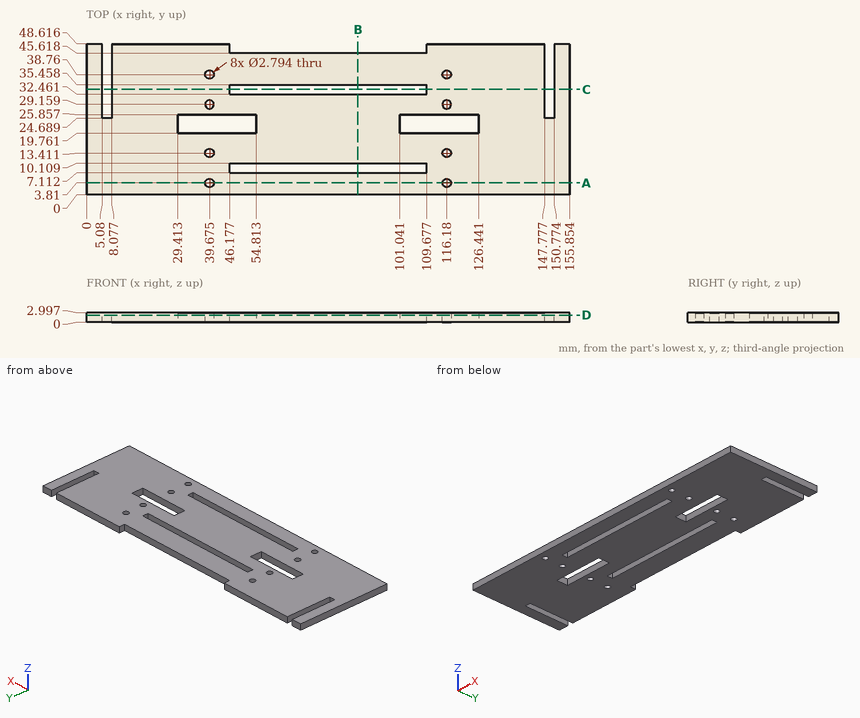
Check sheet for the drawn part. Datum: minimum x, y, z corner. Units: mm. Give positions to 0.01 mm unless a question says otherwise; leave off trailing zeros. Loops run counter-clockwise (first coordinate to the right, second up) from the corner with the lowest first, then second, coordinate; pieces in that order, holes last.
1) Sectioned sample at C-C, the plane y = 34. Enter the section's corners in (x, z) (1 decimal).
2) Depth check by flat-ended pin: pin 1 Ø1.5 at (x, z) = (149, 1.5) entering from +Y. Enter the tip coordinate at first touch or a pass-through.
3) Thickness scan on line 1 along X through (y, z) = (26, 2.6) (1 decimal); line 2 along Y through (x, z) = (99.5, 1.7); line 3 along X through (y, z) = (22, 0.8) (1 decimal). Record the ranges inside material, lowest first.
4) Sectioned sample at B-B, the plane x = 87.5. Enter the section's corners in (y, z).
5) Sectioned sample at A-A, the plane y = 3.81. Enter the section's corners in (x, z) (1 decimal).
6) Sectioned sample at D-D, the plane z = 2.2. Count the separate pieces of the cut face and the enclosed holes in it, then the cut area to 3 significant figures.
Answers:
1. outline: (0, 0) - (5.1, 0) - (5.1, 3) - (0, 3) - close; (8.1, 0) - (46.2, 0) - (46.2, 3) - (8.1, 3) - close; (109.7, 0) - (147.8, 0) - (147.8, 3) - (109.7, 3) - close; (150.8, 0) - (155.9, 0) - (155.9, 3) - (150.8, 3) - close
2. pin 1: stops at y = 24.69
3. line 1: x = 0 to 5.1, 8.1 to 147.8, 150.8 to 155.9
3. line 2: y = 0 to 7.11, 10.11 to 32.46, 35.46 to 45.62
3. line 3: x = 0 to 29.4, 54.8 to 101, 126.4 to 155.9
4. outline: (0, 0) - (7.11, 0) - (7.11, 3) - (0, 3) - close; (10.11, 0) - (32.46, 0) - (32.46, 3) - (10.11, 3) - close; (35.46, 0) - (45.62, 0) - (45.62, 3) - (35.46, 3) - close
5. outline: (0, 0) - (38.3, 0) - (38.3, 3) - (0, 3) - close; (41.1, 0) - (114.8, 0) - (114.8, 3) - (41.1, 3) - close; (117.6, 0) - (155.9, 0) - (155.9, 3) - (117.6, 3) - close
6. separate pieces: 1
6. enclosed holes: 12
6. area: 6,500 mm2
